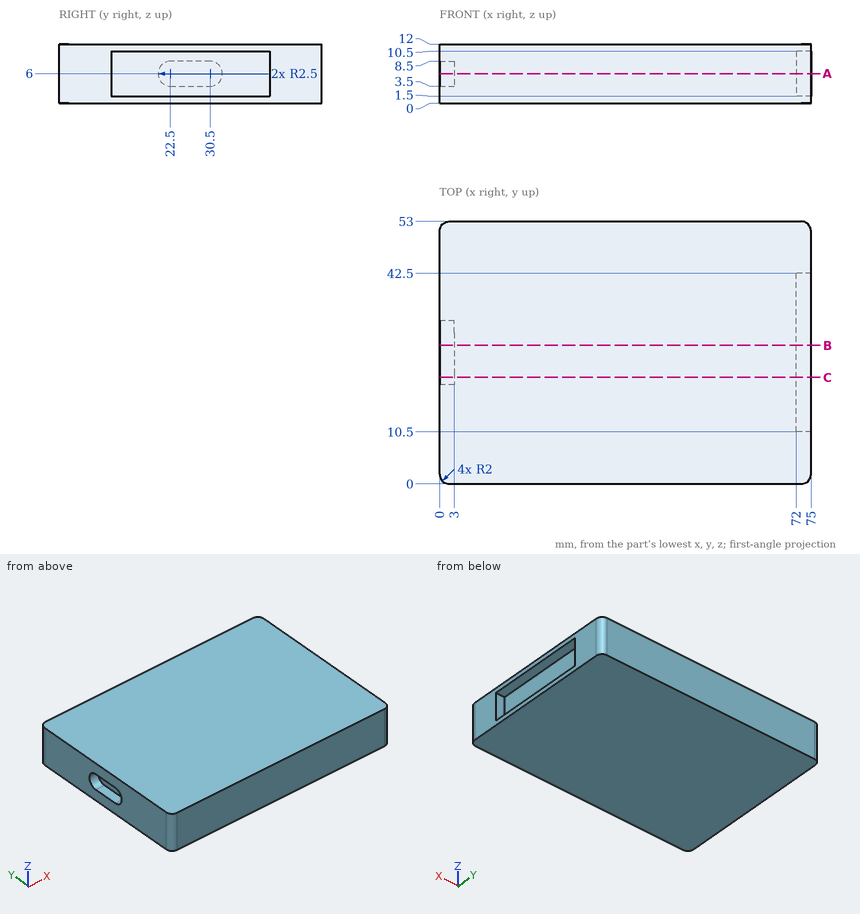
Study the drawing (mm; zero at the part's minimum x, y, z) and answer. Coordinates: 2 decimals unless noted, no trailing zeros. Write each loop counter-clockwise with the first axis right and the second up, starting at its lowest first coordinate (ties: lowest second). Pieces come first, ordered by that corner, then holes. Notation, with made-up numbers: (36.5, 30) - (74.5, 30) arc R29 cw to (74.5, 56) - close; hole circle Ø10 at (61, 73.25). An arc over 180 degrees is marked (long way). Return JSON: item names as keys, results as strings. Group by question number.
1. A cutting plane is placed at B-B, the plane y = 28. Determine the outline of the cut face in (x, z).
2. Straight lines are drawn through the part: L1, parallel to X at y = 34, z = 2; L2, parallel to X at y = 28.5, z = 7. For each, find the intervals that lie inside material, in ascending order.
3. Given pin 1 (5 mm diameter, centred on y = 29.5, z = 6, fed in from +X); pin 2 (1.5 mm diameter, centred on y = 28.5, z = 7, fed in from -X); pin 3 (0.9 mm diameter, centred on x = 74, z = 5, fed in from +Y), each flat-ended and moving along its own axis, determine where each tip first touches the part or whether it passes through.
4. A cutting plane is placed at A-A, the plane z = 6. Determine the outline of the cut face in (x, y), plus the area to 3 significant figures.
5. A cutting plane is placed at C-C, the plane y = 21.5. Determine the outline of the cut face in (x, z).
Ans:
{
 "1": {"outline": "(0, 0) - (75, 0) - (75, 1.5) - (72, 1.5) - (72, 10.5) - (75, 10.5) - (75, 12) - (0, 12) - (0, 8.5) - (3, 8.5) - (3, 3.5) - (0, 3.5) - close"},
 "2": {"L1": "0 to 72", "L2": "3 to 72"},
 "3": {"pin 1": "x = 72", "pin 2": "x = 3", "pin 3": "y = 52.92"},
 "4": {"outline": "(0, 2) arc R2 ccw to (2, 0) - (73, 0) arc R2 ccw to (75, 2) - (75, 10.5) - (72, 10.5) - (72, 42.5) - (75, 42.5) - (75, 51) arc R2 ccw to (73, 53) - (2, 53) arc R2 ccw to (0, 51) - (0, 33) - (3, 33) - (3, 20) - (0, 20) - close", "area": "3,840 mm²"},
 "5": {"outline": "(0, 0) - (75, 0) - (75, 1.5) - (72, 1.5) - (72, 10.5) - (75, 10.5) - (75, 12) - (0, 12) - (0, 8.29) - (3, 8.29) - (3, 3.71) - (0, 3.71) - close"}
}
